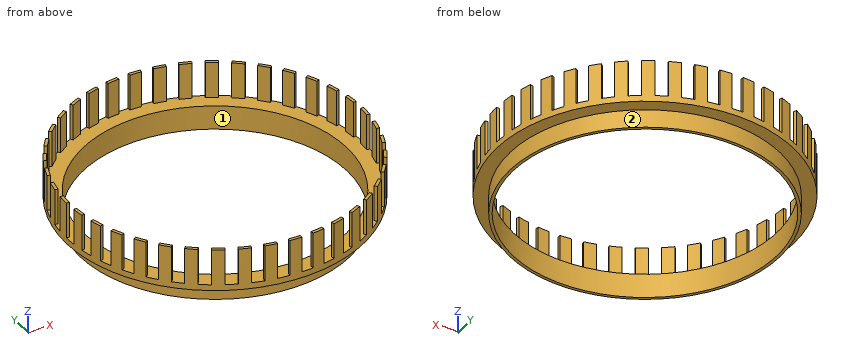
from build123d import *

# Parameters (mm, degrees)
SKETCH_R           = 22.5
SKETCH_R_2         = 22
PAD_DEPTH          = 3
SKETCH001_R        = 24.75
SKETCH001_R_2      = 22
PAD001_DEPTH       = 1
SKETCH002_R        = 24.75
SKETCH002_R_2      = 24.25
PAD002_DEPTH       = 6
POCKET_DEPTH       = 6
POLARPATTERN_COUNT = 40


with BuildPart() as part:
    # Sketch → Pad (new body)
    with BuildSketch(Plane.XY):
        Circle(SKETCH_R)
        Circle(SKETCH_R_2, mode=Mode.SUBTRACT)
    extrude(amount=PAD_DEPTH)

    # Sketch001 (on Face4 of Pad) → Pad001 (join)
    with BuildSketch(Plane.XY.offset(3)):
        Circle(SKETCH001_R)
        Circle(SKETCH001_R_2, mode=Mode.SUBTRACT)
    extrude(amount=PAD001_DEPTH)

    # Sketch002 (on Face5 of Pad001) → Pad002 (join)
    with BuildSketch(Plane.XY.offset(4)):
        Circle(SKETCH002_R)
        Circle(SKETCH002_R_2, mode=Mode.SUBTRACT)
    extrude(amount=PAD002_DEPTH)

    # Sketch003 (on Face7 of Pad002) → Pocket (cut)
    with BuildSketch(Plane.XY.offset(10)):
        with BuildLine():
            ThreePointArc((20.687132, 0), (20.671183, 0.812175), (20.62336, 1.623097))
            Line((20.62336, 1.623097), (25.593958, 2.014293))
            ThreePointArc((25.6731, 0), (25.653307, 1.007924), (25.593958, 2.014293))
            Line((20.687132, 0), (25.6731, 0))
        make_face()
    pocket = extrude(amount=-POCKET_DEPTH, mode=Mode.SUBTRACT)

    # PolarPattern: Pocket ×40 about axis
    polarpattern_axis = Axis((0, 0, 10), (0, 0, 1))
    for i in range(1, POLARPATTERN_COUNT):
        add(pocket.rotate(polarpattern_axis, i * 360 / POLARPATTERN_COUNT), mode=Mode.SUBTRACT)


solid = part.part
Geometry check sheet. Reference: the model listing, model coordinates, mm. Face numbers are marked on the shaded views. Give positions to 0.01 mm unless a question says otherwise; leave off trailing zeros. Order: outer loops, then holes, each group sorted by start corner. A loop starts at its lowest first (then second) coordinate and runs counter-clockwise, first axis right, second up.
1. Scan lines: line 1 (Y direction, x = 0, z = 3.25); line 2 (X direction, y = 0.5, z = 2); line 3 (Z direction, x = -7.5, y = -21). Record each from-to range of solid material in increasing order.
Completed:
line 1: y = -24.75 to -22, 22 to 24.75
line 2: x = -22.49 to -21.99, 21.99 to 22.49
line 3: z = 0 to 4
2. Sectioned sample at B-B (z = 8.75). State how many separate pieces and enclosed holes the cut face has, then the cut area to 3 significant figures.
Completed:
separate pieces: 40
enclosed holes: 0
area: 38.5 mm2
3. Sectioned sample at C-C (z = 1.5). Record the boundary of the cut face in (x, y), then the cut area to 3 significant figures.
Completed:
outline: circle Ø45 at (0, 0); hole circle Ø44 at (0, 0)
area: 69.9 mm2
4. Draft check along Y on the marked faces 1 and 2. Enter one of: pulls with the +Y half, pulls with the -Y half, needs draft (parallel to the pull), parting line crosses it, or undercut.
Completed:
face 1: undercut
face 2: parting line crosses it
5. Depth check by flat-ended pin: pin 1 (1.5 mm diameter, centred on y = -14.5, z = 6.5, fed in from +X); pin 2 (3 mm diameter, centred on x = 6.5, z = 6, fed in from +Y); pin 3 (0.6 mm diameter, centred on y = 24.5, z = 8.5, fed in from -X); pin 4 (15 mm diameter, centred on x = 10, y = -3, fed in from +Z). Enter the tip coordinate at first touch or a pass-through.
Completed:
pin 1: stops at x = 20.02
pin 2: stops at y = 24.24
pin 3: stops at x = -3.87
pin 4: passes through
6. Sectioned sample at A-A (y = 6.5). Record the boundary of the cut face in (x, z).
Completed:
outline: (-23.88, 3) - (-21.54, 3) - (-21.54, 0) - (-21.02, 0) - (-21.02, 4) - (-23.88, 4) - close; (21.02, 0) - (21.54, 0) - (21.54, 3) - (23.88, 3) - (23.88, 10) - (23.36, 10) - (23.36, 4) - (21.02, 4) - close
